from build123d import *

# Parameters (mm, degrees)
SKETCH1_R                = 68.369999998
SKETCH1_R_2              = 62.369999998
BOSS_EXTRUDE1_DEPTH      = 30
SKETCH68_R               = 68.369999998
SKETCH68_R_2             = 66.369999998
BOSS_EXTRUDE2_DEPTH      = 20
CUT_EXTRUDE8_START       = -0.5
SKETCH69_R               = 66.369999998
SKETCH69_R_2             = 64.369999998
CUT_EXTRUDE8_DEPTH       = 0.5
SKETCH72_W               = 10
SKETCH72_H               = 15
CUT_EXTRUDE9_DEPTH       = 129.553881543
CUT_EXTRUDE12_DEPTH      = 122.552738517
CUT_EXTRUDE12_DEPTH_BACK = 122.552738517
SKETCH75_R               = 2
CUT_EXTRUDE13_DEPTH      = 127.128190531
CUT_EXTRUDE13_DEPTH_BACK = 127.128190531
SKETCH76_R               = 2.000000001


with BuildPart() as part:
    # Sketch1 → Boss-Extrude1 (new body)
    with BuildSketch(Plane(origin=(0, 0, 0), x_dir=(-0.9985653746512714, 0, -0.053546172109368295), z_dir=(0, 1, 0))):
        with Locations(Location((29.226008494, -15.877583489, 0), (0, 0, 93.069437642))):
            Circle(SKETCH1_R)
        with Locations(Location((29.226008494, -15.877583489, 0), (0, 0, 93.069437642))):
            Circle(SKETCH1_R_2, mode=Mode.SUBTRACT)
    extrude(amount=BOSS_EXTRUDE1_DEPTH)

    # Sketch68 → Boss-Extrude2 (add)
    with BuildSketch(Plane(origin=(0, 30, 0), x_dir=(1, 0, 0), z_dir=(0, 1, 0))):
        with Locations(Location((-28.333896303, 17.419745986, 0), (0, 0, 270))):
            Circle(SKETCH68_R)
        with Locations(Location((-28.333896303, 17.419745986, 0), (0, 0, 270))):
            Circle(SKETCH68_R_2, mode=Mode.SUBTRACT)
    extrude(amount=BOSS_EXTRUDE2_DEPTH)

    # Sketch69 → Cut-Extrude8 (cut)
    with BuildSketch(Plane(origin=(0, 30, 0), x_dir=(1, 0, 0), z_dir=(0, 1, 0)).offset(CUT_EXTRUDE8_START)):
        with Locations(Location((-28.333896303, 17.419745986, 0), (0, 0, 270))):
            Circle(SKETCH69_R)
        with Locations(Location((-28.333896303, 17.419745986, 0), (0, 0, 270))):
            Circle(SKETCH69_R_2, mode=Mode.SUBTRACT)
    extrude(amount=CUT_EXTRUDE8_DEPTH, mode=Mode.SUBTRACT)

    # Sketch72 → Cut-Extrude9 (cut, through all)
    with BuildSketch(Plane(origin=(0, 0, -17.419745986), x_dir=(-1, 0, 0), z_dir=(0, 0, -1))):
        with Locations((28.333896303, 7.5)):
            Rectangle(SKETCH72_W, SKETCH72_H)
    extrude(amount=-CUT_EXTRUDE9_DEPTH, mode=Mode.SUBTRACT)

    # Sketch75 → Cut-Extrude12 (cut, two sides: drawn at the far end of the back side and taken through both)
    with BuildSketch(Plane(origin=(-27.926429367, 72.899932993, -17.0123656), x_dir=(0.7071818832479886, 0, 0.7070316711476428), z_dir=(-0.7070316711476428, 0, 0.7071818832479886)).offset(-CUT_EXTRUDE12_DEPTH_BACK)):
        with Locations(Location((-0.576184071, -34.599932993, 0), (0, 0, 180))):
            Circle(SKETCH75_R)
    extrude(amount=CUT_EXTRUDE12_DEPTH + CUT_EXTRUDE12_DEPTH_BACK, mode=Mode.SUBTRACT)

    # Sketch76 → Cut-Extrude13 (cut, two sides: drawn at the far end of the back side and taken through both)
    with BuildSketch(Plane(origin=(-32.743645602, 72.899932993, -13.009059816), x_dir=(0.7070316711476428, 0, -0.7071818832479886), z_dir=(0.7071818832479886, 0, 0.7070316711476428)).offset(-CUT_EXTRUDE13_DEPTH_BACK)):
        with Locations((6.236989769, -34.599932997)):
            Circle(SKETCH76_R)
    extrude(amount=CUT_EXTRUDE13_DEPTH + CUT_EXTRUDE13_DEPTH_BACK, mode=Mode.SUBTRACT)


solid = part.part
Geometry check sheet. Reference: the model listing, model coordinates, mm. A direction names the side the tool comes from. Give positions to 0.01 mm unless a question says otherwise; leave off trailing zeros. Write each loop counter-clockwise with the first axis right and the second up, starting at its lowest first coordinate (ties: lowest second). Pieces come first, ordered by that corner, then holes.
1) Thickness scan on line 1 (X direction, y = 28, z = -15.5); line 2 (X direction, y = 46, z = 37.5); line 3 (Z direction, x = 0.5, y = 42.5). Record the ranges inside material, lowest first.
Values follow:
line 1: x = -96.68 to -90.67, 34.01 to 40.01
line 2: x = -69.06 to -65.6, 8.93 to 12.39
line 3: z = -79.41 to -77.2, 42.36 to 44.57
2) Cross-section at C-C (y = 11). Record the boundary of the cut face in (x, z).
Values follow:
outline: (-33.33, 44.75) - (-33.33, 50.77) arc R68.37 ccw (long way) to (-23.33, 50.77) - (-23.33, 44.75) arc R62.37 cw (long way) to start
3) Go/stop test with flat-tipped pins: pin 1 Ø3 at (y, z) = (11, 46.5) entering from -X; pin 2 Ø6 at (x, y) = (-67, 7) entering from +Z; pin 3 Ø5 at (y, z) = (10.5, 48) entering from +X. Record where each tip stops, or that it passes through.
Values follow:
pin 1: stops at x = -56.23
pin 2: stops at z = 40.91
pin 3: stops at x = -1.58
4) Set-up check for faces 3 (the face through (26.1, 29.5, -52.1)), 4 (the face through (20.4, 39.5, -63.9)), 5 (the face through (-23.334, 7, 48)): record each of +Z, -Z, +X, -X, +Y, -Y from which the full face is reachable in a straight line by a thin tool's end or side.
Values follow:
face 3: +Y
face 4: none
face 5: +Z, -Y
5) Cross-section at B-B (x = -38.5). Record the boundary of the cut face in (y, z).
Values follow:
outline: (0, -85.03) - (50, -85.03) - (50, -83.01) - (29.5, -83.01) - (29.5, -80.98) - (30, -80.98) - (30, -78.96) - (0, -78.96) - close; (0, 44.12) - (30, 44.12) - (30, 46.14) - (29.5, 46.14) - (29.5, 48.17) - (50, 48.17) - (50, 50.19) - (0, 50.19) - close
6) Cross-section at D-D (y = 34.5). Record the boundary of the cut face in (x, z), plus the area to 3 significant figures.
Values follow:
outline: circle Ø136.74 at (-28.33, -17.42); hole circle Ø132.74 at (-28.33, -17.42)
area: 847 mm2
7) Release check for a two-part mould opening along X. For faces 1 (the face through (24.4, 30, -51.1)), 2 (the face through (28, 50, -53)) record: released by +X, released by -X, zero draft, split by the parting line, or undercut.
Values follow:
face 1: undercut
face 2: zero draft
8) Cross-section at A-A (z = -48). Record the boundary of the cut face in (x, y), plus the area to 3 significant figures.
Values follow:
outline: (-89.48, 0) - (-82.69, 0) - (-82.69, 30) - (-84.98, 30) - (-84.98, 29.5) - (-87.24, 29.5) - (-87.24, 50) - (-89.48, 50) - close; (26.02, 0) - (32.82, 0) - (32.82, 50) - (30.57, 50) - (30.57, 29.5) - (28.31, 29.5) - (28.31, 30) - (26.02, 30) - close
area: 495 mm2
